```python
from build123d import *

# Parameters (mm, degrees)
BOSS_EXTRUDE1_DEPTH = 4


with BuildPart() as part:
    # Sketch2 → Loft1 section 0
    with BuildSketch(Plane(origin=(0, 16, 0), x_dir=(1, 0, 0), z_dir=(0, 1, 0))):
        with BuildLine():
            Line((23.69, 0), (11.845, 20.516141816))
            Line((11.845, 20.516141816), (-11.845, 20.516141816))
            Line((-11.845, 20.516141816), (-23.69, 0))
            Line((-23.69, 0), (-11.845, -20.516141816))
            Line((-11.845, -20.516141816), (11.845, -20.516141816))
            Line((11.845, -20.516141816), (23.69, 0))
        make_face()
    # Sketch1 → Loft1 section 1
    with BuildSketch(Plane(origin=(0, 0, 0), x_dir=(1, 0, 0), z_dir=(0, 1, 0))):
        with BuildLine():
            Line((26, 0), (13, 22.516660498))
            Line((13, 22.516660498), (-13, 22.516660498))
            Line((-13, 22.516660498), (-26, 0))
            Line((-26, 0), (-13, -22.516660498))
            Line((-13, -22.516660498), (13, -22.516660498))
            Line((13, -22.516660498), (26, 0))
        make_face()
    loft()

    # Sketch3 → Boss-Extrude1 (add)
    with BuildSketch(Plane(origin=(0, 16, 0), x_dir=(1, 0, 0), z_dir=(0, 1, 0))):
        Polygon((23.69, 0), (11.845, 20.516141816), (-11.845, 20.516141816), (-23.69, 0), (-11.845, -20.516141816), (11.845, -20.516141816), align=None)
    extrude(amount=BOSS_EXTRUDE1_DEPTH)

    # Sketch5 → Cut-Loft1 section 0
    with BuildSketch(Plane(origin=(0, 16, 0), x_dir=(-1, 0, 0), z_dir=(0, -1, 0))):
        with BuildLine():
            Line((20.69, 0), (10.345, 17.918065604))
            Line((10.345, 17.918065604), (-10.345, 17.918065604))
            Line((-10.345, 17.918065604), (-20.69, 0))
            Line((-20.69, 0), (-10.345, -17.918065604))
            Line((-10.345, -17.918065604), (10.345, -17.918065604))
            Line((10.345, -17.918065604), (20.69, 0))
        make_face()
    # Sketch4 → Cut-Loft1 section 1
    with BuildSketch(Plane(origin=(0, -2, 0), x_dir=(-1, 0, 0), z_dir=(0, -1, 0))):
        with BuildLine():
            Line((23, 0), (11.5, 19.918584287))
            Line((11.5, 19.918584287), (-11.5, 19.918584287))
            Line((-11.5, 19.918584287), (-23, 0))
            Line((-23, 0), (-11.5, -19.918584287))
            Line((-11.5, -19.918584287), (11.5, -19.918584287))
            Line((11.5, -19.918584287), (23, 0))
        make_face()
    loft(mode=Mode.SUBTRACT)


solid = part.part
```
Source: CAD feature listing. Evaluate the final solid. Frame: model axes, mm. A direction names the side the tool comes from. Round coordinates to 2 decimals unless told otherwise and drop trailing zeros. Loops run counter-clockwise (first coordinate to the right, second up) from the corner with the lowest first, then second, coordinate; pieces in that order, holes last. Notation, with made-up numbers: M 65.5,-8.5 L 114.5,-8.5 A26 ccw 114.5,7.5 Z; hole C 62.5,-11.75 d4. An arc over 180 degrees is marked long. Use a Markdown table: item, result. Add a question column.
1. Reachability of faces 4 (the flat face through (-17.85, 17.972, 10.114)), 5 (the flat face through (17.685, 17.972, 10.402)), 6 (the flat face through (-17.685, 17.972, -10.402)) from +Z, -Z, +X, -X, +Y, -Y: full face, straight path, thin tool, end or side. Return the list, or none.
2. Contact query for flat-ended pins moving along their axis: P1, Ø12, axis at x = -15.5, y = 8, coming from the -Z side; P2, Ø1.2, axis at x = -0.5, y = 18, coming from the -Z side; P3, Ø1.5, axis at x = -8.5, y = 5.5, coming from the -Z side; P4, Ø10, axis at x = 11, y = 3.5, coming from the +Z side. Output: stop coordinate, or through.
3. Section query A-A on y = 16.75. Return the cut outline in (x, z) (3 decimals).
4. Mould query, pull axis Z, two halves, no side actions, for faces 1 (the flat face through (-17.21, 0, 9.9)), 2 (the flat face through (0, 16, 0)), 3 (the flat face through (17.85, 17.972, -10.114)). Classes: pulls with the +Z half, pulls with the -Z half, needs draft (parallel to the pull), parting line crosses it, or undercut.
5. Line query: line 1 (X direction, y = 16.5, z = 10); line 2 (Y direction, x = -3.5, z = 7); line 3 (Z direction, x = -8.5, y = 5). Output: solid intervals per line, ascending.
Reported:
| question | item | result |
|---|---|---|
| 1 | face 4 | +Z, -X, +Y |
| 1 | face 5 | +Z, +X, +Y |
| 1 | face 6 | -Z, -X, +Y |
| 2 | P1 | stops at z = -22.19 |
| 2 | P2 | stops at z = -20.52 |
| 2 | P3 | stops at z = -21.92 |
| 2 | P4 | stops at z = 22.52 |
| 3 | outline | M -23.69,0 L -11.845,-20.516 L 11.845,-20.516 L 23.69,0 L 11.845,20.516 L -11.845,20.516 Z |
| 4 | face 1 | needs draft |
| 4 | face 2 | undercut |
| 4 | face 3 | pulls with the -Z half |
| 5 | line 1 | x = -17.92 to 17.92 |
| 5 | line 2 | y = 16 to 20 |
| 5 | line 3 | z = -21.89 to -19.14, 19.14 to 21.89 |
